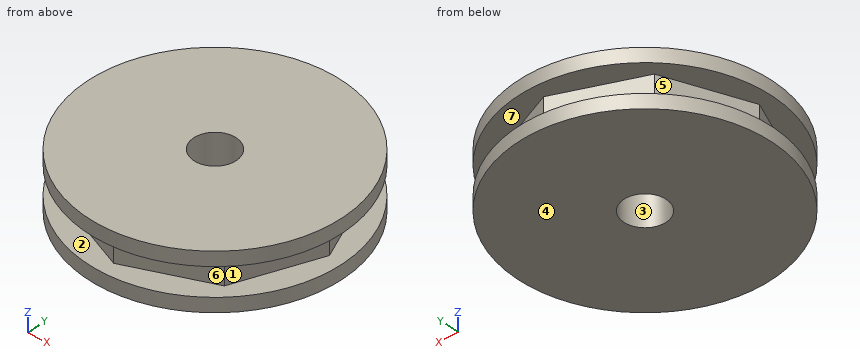
```python
from build123d import *

# Parameters (mm, degrees)
PAD_DEPTH    = 2
SKETCH001_R  = 9
PAD001_DEPTH = 1
SKETCH002_R  = 9
PAD002_DEPTH = 1
SKETCH003_R  = 1.5
POCKET_DEPTH = 5


with BuildPart() as part:
    # Sketch → Pad (new body)
    with BuildSketch(Plane.XY):
        Polygon((0, 8), (-5.656854, 5.656854), (-8, 0), (-5.656854, -5.656854), (0, -8), (5.656854, -5.656854), (8, 0), (5.656854, 5.656854), align=None)
    extrude(amount=PAD_DEPTH)

    # Sketch001 (on Face10 of Pad) → Pad001 (join)
    with BuildSketch(Plane.XY.offset(2)):
        Circle(SKETCH001_R)
    extrude(amount=PAD001_DEPTH)

    # Sketch002 (on Face12 of Pad001) → Pad002 (join)
    with BuildSketch(Plane(origin=(0, 0, 0), x_dir=(1, 0, 0), z_dir=(0, 0, -1))):
        Circle(SKETCH002_R)
    extrude(amount=PAD002_DEPTH)

    # Sketch003 (on Face3 of Pad002) → Pocket (cut)
    with BuildSketch(Plane(origin=(0, 0, -1), x_dir=(1, 0, 0), z_dir=(0, 0, -1))):
        Circle(SKETCH003_R)
    extrude(amount=-POCKET_DEPTH, mode=Mode.SUBTRACT)


solid = part.part
```
Here's how the part is built. I have some questions about the finished solid (model axes, mm). Face numbers are marked on the shaded views. A direction names the side the tool comes from. Round coordinates to 2 decimals unless told otherwise and drop trailing zeros. Order: outer loops, then holes, each group sorted by start corner. A loop starts at its lowest first (then second) coordinate and runs counter-clockwise, first axis right, second up. Notation, with made-up numbers: (-15.75, -10) -> (-5.75, -10) arc R29 ccw to (-5.75, 16) -> close; hole circle Ø10 at (-35.75, 86.5). An arc over 180 degrees is marked (long way). Use a Markdown table: item, result. Add a question column.
(1) Suppose I cut it at D-D, the plane y = -4.25. Please give me the cut outline in (x, z).
(2) Suppose I cut it at B-B, the plane x = -0.5. Please give me the cut outline in (y, z).
(3) Suppose I cut it at A-A, the plane z = 0.75. Please give me the cut outline in (x, y), and give its area (3 significant figures).
(4) For pin 1 Ø2.5 at (x, y) = (0, 0) entering from -Z, with a flat end and sliding along its axis, tell me the tip position at first contact or that it passes through.
(5) For the marked faces 5, 6 and 7, which set-ups out of +Z, -Z, +X, -X, +Y, -Y let a thin tool reach every point of the face, with its end or its side?
(6) Suppose I cut it at C-C, the plane y = 1.25. Please give me the cut outline in (x, z).
(7) I need wall thicknesses on line 1 along Z through (x, y) = (-7, -5.25); line 2 along Y through (x, z) = (0, -0.05); line 3 along Y through (x, z) = (-0.75, 2.2). Which ranges of each line are inside material? Lowest first, please.
(8) If we mould it in two halves opening along Z, with no side actions, what happens to the marked faces 1, 2, 3 and 4? For each: released by +Z, released by -Z, zero draft, split by the parting line, or undercut.
Verdict:
| question | item | result |
|---|---|---|
| 1 | outline | (-7.93, -1) -> (7.93, -1) -> (7.93, 0) -> (6.24, 0) -> (6.24, 2) -> (7.93, 2) -> (7.93, 3) -> (-7.93, 3) -> (-7.93, 2) -> (-6.24, 2) -> (-6.24, 0) -> (-7.93, 0) -> close |
| 2 | outline | (-8.99, -1) -> (-1.41, -1) -> (-1.41, 3) -> (-8.99, 3) -> (-8.99, 2) -> (-7.79, 2) -> (-7.79, 0) -> (-8.99, 0) -> close; (1.41, -1) -> (8.99, -1) -> (8.99, 0) -> (7.79, 0) -> (7.79, 2) -> (8.99, 2) -> (8.99, 3) -> (1.41, 3) -> close |
| 3 | outline | (-8, 0) -> (-5.66, -5.66) -> (0, -8) -> (5.66, -5.66) -> (8, 0) -> (5.66, 5.66) -> (0, 8) -> (-5.66, 5.66) -> close; hole circle Ø3 at (0, 0) |
| 3 | area | 174 mm2 |
| 4 | pin 1 | through |
| 5 | face 5 | -X, +Y |
| 5 | face 6 | +X, -Y |
| 5 | face 7 | none |
| 6 | outline | (-8.91, -1) -> (-0.83, -1) -> (-0.83, 3) -> (-8.91, 3) -> (-8.91, 2) -> (-7.48, 2) -> (-7.48, 0) -> (-8.91, 0) -> close; (0.83, -1) -> (8.91, -1) -> (8.91, 0) -> (7.48, 0) -> (7.48, 2) -> (8.91, 2) -> (8.91, 3) -> (0.83, 3) -> close |
| 7 | line 1 | -1 to 0, 2 to 3 |
| 7 | line 2 | -9 to -1.5, 1.5 to 9 |
| 7 | line 3 | -8.97 to -1.3, 1.3 to 8.97 |
| 8 | face 1 | undercut |
| 8 | face 2 | undercut |
| 8 | face 3 | zero draft |
| 8 | face 4 | released by -Z |
